For this review, take the finished solid that the model builds, in its own axes (mm). A direction names the side the tool comes from. Coordinates: 2 decimals unless noted, no trailing zeros. Loops run counter-clockwise (first coordinate to the right, second up) from the corner with the lowest first, then second, coordinate; pieces in that order, holes last. Notation, with made-up numbers: (42, 35) -> (94, 35) arc R26 cw to (94, 53) -> close; hole circle Ø1 at (36, 85.5). An arc over 180 degrees is marked (long way). Answer in a Markdown table with one row per item.
Autodesk Inventor part; units mm, degrees
ref_plane "YZ Plane" through (0, 0, 0) normal (1, 0, 0) x (0, 1, 0)
ref_plane "XZ Plane" through (0, 0, 0) normal (0, 1, 0) x (-1, 0, 0)
ref_plane "XY Plane" through (0, 0, 0) normal (0, 0, 1) x (1, 0, 0)
sketch "Sketch1" plane through (0, 0, 0) normal (0, 0, 1) x (1, 0, 0)
  arc A0 (0, 3.175) -> (-3.175, 0) centre (0, 0) ccw
  arc A1 (-3.175, -22.86) -> (0, -26.035) centre (0, -22.86) ccw
  line L0 (0, -26.035) -> (27.94, -26.035)
  line L1 (0, 3.175) -> (27.94, 3.175)
  circle A2 centre (0, -22.86) radius 1.5875
  circle A3 centre (27.94, -22.86) radius 1.5875
  circle A4 centre (0, 0) radius 1.5875
  circle A5 centre (27.94, 0) radius 1.5875
  arc A6 (-3.175, -22.86) -> (-3.175, 0) centre (-101.9139, -11.43) ccw
  arc A7 (31.115, 0) -> (31.115, -22.86) centre (133.6675, -11.43) ccw
  arc A8 (27.94, -26.035) -> (31.115, -22.86) centre (27.94, -22.86) ccw
  arc A9 (31.115, 0) -> (27.94, 3.175) centre (27.94, 0) ccw
  point P0 (30.48, -11.43)
  point P1 (-2.54, -11.43)
  point P2 (-3.0961, -0.7033)
  dimension "d0" = 27.94
  dimension "d1" = 22.86
  dimension "d3" = 6.35
  dimension "d4" = 6.35
  dimension "d6" = 33.02
  dimension "d7" = 11.43
  dimension "d8" = 2.54
  dimension "d9" = 3.175
  dimension "d10" = 3.175
  dimension "d11" = 3.175
  dimension "d12" = 3.175
  dimension "d34" = 27.94
  dimension "d35" = 22.86
  dimension "d36" = 0
  dimension "d37" = 0
extrude "Extrusion1" add sketch "Sketch1" along normal blind 1.27
sketch "Sketch2" plane through (0, 0, 1.27) normal (0, 0, 1) x (1, 0, 0)
  circle A0 centre (13.97, -11.43) radius 13.335
  point P0 (0, 0)
  dimension "d15" = 26.67
  dimension "d16" = 13.97
  dimension "d17" = 11.43
extrude "Extrusion2" add sketch "Sketch2" along normal blind 10.16
sketch "Sketch3" plane through (13.97, -11.43, 11.43) normal (0, 0, 1) x (1, 0, 0)
  line L0 (9.525, -5.08) -> (10.795, -5.08)
  line L1 (10.795, -5.08) -> (10.795, -17.78)
  line L2 (10.795, -17.78) -> (9.525, -17.78)
  line L3 (9.525, -17.78) -> (9.525, -5.08)
  line L4 (-10.795, -5.08) -> (-9.525, -5.08)
  line L5 (-9.525, -5.08) -> (-9.525, -17.78)
  line L6 (-9.525, -17.78) -> (-10.795, -17.78)
  line L7 (-10.795, -17.78) -> (-10.795, -5.08)
  circle A0 centre (0, 0) radius 13.335
  point P0 (-13.97, 11.43)
  point P1 (-13.335, 0)
  dimension "d20" = 19.05
  dimension "d21" = 1.27
  dimension "d22" = 1.27
  dimension "d23" = 3.81
  dimension "d24" = 5.08
  dimension "d25" = 12.7
extrude "Extrusion3" add sketch "Sketch3" along normal blind 17.78 contours L0 L1 A0 L3 | A0 L1 L2 L3 | A0 L7 L4 L5 | L5 L6 L7 A0
sketch "Sketch4" plane through (24.765, -29.21, 11.43) normal (1, 0, 0) x (0, 0, -1)
  line L0 (0, 0) -> (-17.78, 0)
  line L1 (-17.78, 0) -> (-17.78, 12.7)
  circle A0 centre (-12.7, 5.08) radius 1.5875
  point P0 (11.43, 29.21)
  dimension "d28" = 5.08
  dimension "d29" = 5.08
  dimension "d30" = 3.175
extrude "Extrusion4" cut sketch "Sketch4" against normal blind 50.8
fillet "Fillet1" radius 5.08 8 edges at (24.13, -29.21, 29.21) (3.81, -29.21, 29.21) (24.13, -16.51, 29.21) (3.81, -16.51, 29.21) (3.81, -16.51, 11.43) (24.13, -16.51, 11.43) (3.81, -29.21, 11.43) (24.13, -29.21, 11.43)
properties part number "CastorBase" material "Stainless Steel"
Item 1: For L1, parallel to Y at x = 27.94, z = 0.5 (1 decimal); L2, parallel to Y at x = 3.65, z = 24.13; L3, parallel to X at y = -20, z = 21.75 (3 decimals), list the stretches that pass through material, from the lowest coordinate up.
Worked answers:
| item | result |
|---|---|
| L1 | -26 to -24.4, -21.3 to -1.6, 1.6 to 3.2 |
| L2 | -29.21 to -25.72, -22.54 to -16.51 |
| L3 | 3.175 to 4.445, 23.495 to 24.765 |
Item 2: Take a section at A-A, the plane z = 20.75. State the section outline as (x, y) points (3 decimals).
Worked answers:
| item | result |
|---|---|
| outline | (3.175, -29.21) -> (4.445, -29.21) -> (4.445, -16.51) -> (3.175, -16.51) -> close; (23.495, -29.21) -> (24.765, -29.21) -> (24.765, -16.51) -> (23.495, -16.51) -> close |
Item 3: For faces 4 (the flat face through (23.495, -22, 20)), 5 (the flat face through (24.765, -22, 20)), 6 (the flat face through (4, -22, 11.43)), 7 (the flat face through (14, 3.175, 1)), 8 (the flat face through (3.175, -22, 20)), list the 3-axis set-ups (+Z, -Z, +X, -X, +Y, -Y) from which the entire face can be reached by the end or side of a thin tool; tool diameter is ignored.
Worked answers:
| item | result |
|---|---|
| face 4 | +Z, +Y, -Y |
| face 5 | +Z, +X, +Y, -Y |
| face 6 | -X, -Y |
| face 7 | +Z, -Z, +X, -X, +Y |
| face 8 | +Z, -X, +Y, -Y |
Item 4: Take a section at B-B, the plane x = -0.5. State the section outline as (y, z) points.
Worked answers:
| item | result |
|---|---|
| outline | (-26, 0) -> (-24.37, 0) -> (-24.37, 1.27) -> (-26, 1.27) -> close; (-21.35, 0) -> (-1.51, 0) -> (-1.51, 1.27) -> (-21.35, 1.27) -> close; (1.51, 0) -> (3.14, 0) -> (3.14, 1.27) -> (1.51, 1.27) -> close |
Item 5: The part is to be moulded in two halves that separate along Y. For faces 1 (the cylindrical face through (3.82, -22.79, 23.28)), 2 (the flat face through (2, -5, 1.27)), 3 (the cylindrical face through (30.21, -25.08, 0.63)), say which applies: +Y half, -Y half, draft (parallel to the pull), parting line (faces both ways), or undercut.
Worked answers:
| item | result |
|---|---|
| face 1 | undercut |
| face 2 | draft |
| face 3 | -Y half |
Item 6: Take a section at C-C, the plane y = -16. State the section outline as (x, z) points (3 decimals), and give its area (3 significant figures).
Worked answers:
| item | result |
|---|---|
| outline | (-2.621, 0) -> (30.581, 0) -> (30.581, 1.27) -> (26.497, 1.27) -> (26.497, 11.43) -> (24.765, 11.43) -> (24.765, 14.292) -> (23.495, 14.292) -> (23.495, 11.43) -> (4.445, 11.43) -> (4.445, 14.292) -> (3.175, 14.292) -> (3.175, 11.43) -> (1.443, 11.43) -> (1.443, 1.27) -> (-2.621, 1.27) -> close |
| area | 304 mm² |
Item 7: Insertion check: pin 1 (3.5 mm diameter, centred on y = -24.13, z = 24.13, fed in from +X) (3 decimals); pin 2 (1 mm diameter, centred on x = 4, z = 19.5, fed in from +Y); pin 3 (1.5 mm diameter, centred on y = -5, z = 9.5, fed in from +X). Each pin has a flat end and moves straight along its axis. Give the tip position at first contact, or say it passes through.
Worked answers:
| item | result |
|---|---|
| pin 1 | x = 24.765 |
| pin 2 | y = -16.51 |
| pin 3 | x = 26.03 |
Item 8: Take a section at D-D, the plane x = 7. State the section outline as (y, z) points (3 decimals), and give its area (3 significant figures).
Worked answers:
| item | result |
|---|---|
| outline | (-26.035, 0) -> (3.175, 0) -> (3.175, 1.27) -> (-0.062, 1.27) -> (-0.062, 11.43) -> (-22.798, 11.43) -> (-22.798, 1.27) -> (-26.035, 1.27) -> close |
| area | 268 mm² |
